Read the model definition and answer for the solid it produces. Units are mm, in the model's axes. Face numbers are marked on the shaded views. A direction names the side the tool comes from. Coordinates: 2 decimals unless noted, no trailing zeros. Order: outer loops, then holes, each group sorted by start corner. A loop starts at its lowest first (then second) coordinate and runs counter-clockwise, first axis right, second up. Notation, with made-up numbers: (61.5, 81.5) -> (93.5, 81.5) arc R35 ccw to (93.5, 120.5) -> close; hole circle Ø2 at (-33, -3.5). An arc over 180 degrees is marked (long way). Answer in a Markdown table with one row per item.
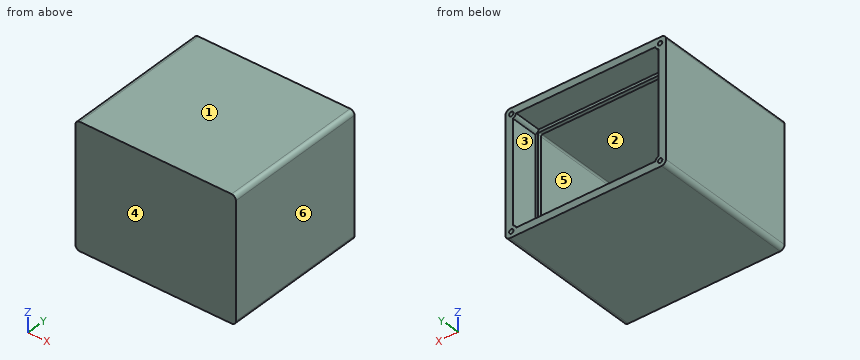
from build123d import *

# Parameters (mm, degrees)
SKETCH1_W                = 100
SKETCH1_H                = 75
BOSS_EXTRUDE1_DEPTH      = 95
SHELL1_T                 = 5
FILLET2_R                = 3
SKETCH6_R                = 3.5
BOSS_EXTRUDE4_DEPTH      = 19
SKETCH6_4_R              = 1.5
CUT_EXTRUDE2_DEPTH       = 15
FILLET3_R                = 1
BOSS_EXTRUDE5_DEPTH      = 1
BOSS_EXTRUDE5_DEPTH_BACK = 1.5
SKETCH8_W                = 100
SKETCH8_H                = 75
SKETCH8_W_2              = 96
SKETCH8_H_2              = 71
FILLET4_R                = 1


with BuildPart() as part:
    # Sketch1 → Boss-Extrude1 (new body)
    with BuildSketch(Plane(origin=(0, 0, 0), x_dir=(1, 0, 0), z_dir=(0, 1, 0))):
        with Locations((50, 37.5)):
            Rectangle(SKETCH1_W, SKETCH1_H)
    extrude(amount=BOSS_EXTRUDE1_DEPTH)

    # Shell1
    shell1_openings = [part.faces().sort_by_distance(p)[0] for p in [
        (50, 95, -37.5),
    ]]
    offset(amount=SHELL1_T, openings=shell1_openings, kind=Kind.INTERSECTION)

    # Fillet2
    # the kernel refuses this fillet: 3 mm, written as the material it takes off along each edge
    with BuildSketch(Plane(origin=(-5, -12.5, -80), x_dir=(1, 0, 0), z_dir=(0, 1, 0)), Plane(origin=(105, -12.5, -80), x_dir=(0, 0, 1), z_dir=(0, 1, 0)), Plane(origin=(105, -12.5, 5), x_dir=(-1, 0, 0), z_dir=(0, 1, 0)), Plane(origin=(-5, 102.5, 5), x_dir=(1, 0, 0), z_dir=(0, -1, 0))) as fillet2_piece_1:
        with BuildLine():
            CenterArc((FILLET2_R, -FILLET2_R), FILLET2_R, 90, 90)
            Line((0, -FILLET2_R), (0, 0))
            Line((0, 0), (FILLET2_R, 0))
        make_face()
    extrude(amount=115, mode=Mode.SUBTRACT)

    # Sketch6 → Boss-Extrude4 (add)
    with BuildSketch(Plane(origin=(0, 95, 0), x_dir=(1, 0, 0), z_dir=(0, 1, 0))):
        with Locations((-1, 76)):
            Circle(SKETCH6_R)
        with Locations((101, 76)):
            Circle(SKETCH6_R)
        with Locations((101, -1)):
            Circle(SKETCH6_R)
        with Locations((-1, -1)):
            Circle(SKETCH6_R)
    extrude(amount=-BOSS_EXTRUDE4_DEPTH)

    # Sketch6<4> → Cut-Extrude2 (cut)
    with BuildSketch(Plane(origin=(0, 95, 0), x_dir=(1, 0, 0), z_dir=(0, 1, 0))):
        with Locations(Location((-1, 76, 0), (0, 0, 270))):
            Circle(SKETCH6_4_R)
        with Locations(Location((101, 76, 0), (0, 0, 90))):
            Circle(SKETCH6_4_R)
        with Locations(Location((101, -1, 0), (0, 0, 270))):
            Circle(SKETCH6_4_R)
        with Locations(Location((-1, -1, 0), (0, 0, 90))):
            Circle(SKETCH6_4_R)
    extrude(amount=-CUT_EXTRUDE2_DEPTH, mode=Mode.SUBTRACT)

    # Fillet3
    fillet3_edges = [part.edges().sort_by_distance(p)[0] for p in [
        (0, 38, 0),
        (0, 38, -75),
        (100, 38, -75),
        (100, 38, 0),
    ]]
    fillet(fillet3_edges, radius=FILLET3_R)

    # Sketch8 → Boss-Extrude5 (add, two sides: drawn at the far end of the back side and taken through both)
    with BuildSketch(Plane(origin=(0, 75, 0), x_dir=(1, 0, 0), z_dir=(0, 1, 0)).offset(-BOSS_EXTRUDE5_DEPTH_BACK)):
        with Locations((50, 37.5)):
            Rectangle(SKETCH8_W, SKETCH8_H)
        with Locations((50, 37.5)):
            Rectangle(SKETCH8_W_2, SKETCH8_H_2, mode=Mode.SUBTRACT)
    extrude(amount=BOSS_EXTRUDE5_DEPTH + BOSS_EXTRUDE5_DEPTH_BACK)

    # Fillet4
    fillet4_edges = [part.edges().sort_by_distance(p)[0] for p in [
        (2, 74.75, -73),
        (98, 74.75, -73),
        (98, 74.75, -2),
        (2, 74.75, -2),
    ]]
    fillet(fillet4_edges, radius=FILLET4_R)


solid = part.part
Q1. For the marked faces 1, 2 and 3, determine the directions among +Z, -Z, +X, -X, +Y, -Y from which every point of the face is accessible in a straight line to the end or side of a thin tool.
Outcome:
| item | result |
|---|---|
| face 1 | +Z, +X, -X, +Y, -Y |
| face 2 | none |
| face 3 | +Y |
Q2. The part is cut by section A-A (y = 60). Write down the section's boundary in (x, z), then the cut area to 3 significant figures.
Outcome:
| item | result |
|---|---|
| outline | (-5, -77) arc R3 ccw to (-2, -80) -> (102, -80) arc R3 ccw to (105, -77) -> (105, 2) arc R3 ccw to (102, 5) -> (-2, 5) arc R3 ccw to (-5, 2) -> close; hole (0, -74) arc R1 ccw to (1, -75) -> (99, -75) arc R1 ccw to (100, -74) -> (100, -1) arc R1 ccw to (99, 0) -> (1, 0) arc R1 ccw to (0, -1) -> close |
| area | 1,840 mm² |
Q3. The part is cut by section B-B (z = -66). Write down the section's boundary in (x, y).
Outcome:
| item | result |
|---|---|
| outline | (-5, -5) -> (105, -5) -> (105, 95) -> (100, 95) -> (100, 76) -> (98, 76) -> (98, 73.5) -> (100, 73.5) -> (100, 0) -> (0, 0) -> (0, 73.5) -> (2, 73.5) -> (2, 76) -> (0, 76) -> (0, 95) -> (-5, 95) -> close |
Q4. For a pull along Y with two mould halves and no side action, classify the marked faces 4, 5 and 6 as pulls with the +Y half, pulls with the -Y half, needs draft (parallel to the pull), parting line crosses it, or undercut.
Outcome:
| item | result |
|---|---|
| face 4 | pulls with the -Y half |
| face 5 | undercut |
| face 6 | needs draft |
Q5. Consider line 1 (Z direction, x = 101, y = 84.75); line 2 (X direction, y = 84.75, z = -76); line 3 (X direction, y = 55.5, z = -69.5). Determine where each line is inside the solid, lowest interval first.
Outcome:
| item | result |
|---|---|
| line 1 | -80 to -77.5, -74.5 to -0.5, 2.5 to 5 |
| line 2 | -5 to -2.5, 0.5 to 99.5, 102.5 to 105 |
| line 3 | -5 to 0, 100 to 105 |
Q6. The part is cut by section C-C (x = 44.5). Write down the section's boundary in (y, z).
Outcome:
| item | result |
|---|---|
| outline | (-5, -80) -> (95, -80) -> (95, -75) -> (76, -75) -> (76, -73) -> (73.5, -73) -> (73.5, -75) -> (0, -75) -> (0, 0) -> (73.5, 0) -> (73.5, -2) -> (76, -2) -> (76, 0) -> (95, 0) -> (95, 5) -> (-5, 5) -> close |
Q7. Given pin 1 (8 mm diameter, centred on x = 18, z = -55, fed in from +Y); pin 2 (1.8 mm diameter, centred on x = -1, z = -76, fed in from +Y), each flat-ended and moving along its own axis, determine where each tip first touches the part or whether it passes through.
Outcome:
| item | result |
|---|---|
| pin 1 | y = 0 |
| pin 2 | y = 80 |
